Here's how the part is built. I have some questions about the finished solid (model axes, mm). Face numbers are marked on the shaded views. A direction names the side the tool comes from. Round coordinates to 2 decimals unless told otherwise and drop trailing zeros. Loops run counter-clockwise (first coordinate to the right, second up) from the corner with the lowest first, then second, coordinate; pieces in that order, holes last. Notation, with made-up numbers: M -21,-26.75 L 18,-26.75 A23 cw 18,-13.75 Z; hole C 33.5,-3.5 d4. An arc over 180 degrees is marked long. One line per question, with ' | ' between items. Start each with the question number.
```python
from build123d import *

# Parameters (mm, degrees)
BOSS_EXTRUDE1_DEPTH = 3
BOSS_EXTRUDE3_DEPTH = 3


with BuildPart() as part:
    # Sketch1 → Boss-Extrude1 (new body)
    with BuildSketch(Plane(origin=(0, 0, 0), x_dir=(1, 0, 0), z_dir=(0, 1, 0))):
        with BuildLine():
            Line((0, -6.1), (-30, -6.1))
            ThreePointArc((-30, -6.1), (-36.1, 0), (-30, 6.1))
            Line((-30, 6.1), (0, 6.1))
            Line((0, 6.1), (0, -6.1))
        make_face()
        with BuildLine():
            Line((-30, 3.1), (-25, 3.1))
            ThreePointArc((-25, 3.1), (-21.9, 0), (-25, -3.1))
            Line((-25, -3.1), (-30, -3.1))
            ThreePointArc((-30, -3.1), (-33.1, 0), (-30, 3.1))
        make_face(mode=Mode.SUBTRACT)
    extrude(amount=BOSS_EXTRUDE1_DEPTH)

    # Sketch4 → Boss-Extrude3 (add)
    with BuildSketch(Plane(origin=(0, 0, 0), x_dir=(0, 0, -1), z_dir=(1, 0, 0))):
        with BuildLine():
            Line((-6.1, 0), (-6.1, 30))
            ThreePointArc((-6.1, 30), (0, 36.1), (6.1, 30))
            Line((6.1, 30), (6.1, 0))
            Line((6.1, 0), (-6.1, 0))
        make_face()
        with BuildLine():
            Line((3.1, 30), (3.1, 25))
            ThreePointArc((3.1, 25), (0, 21.9), (-3.1, 25))
            Line((-3.1, 25), (-3.1, 30))
            ThreePointArc((-3.1, 30), (0, 33.1), (3.1, 30))
        make_face(mode=Mode.SUBTRACT)
    extrude(amount=-BOSS_EXTRUDE3_DEPTH)


solid = part.part
```
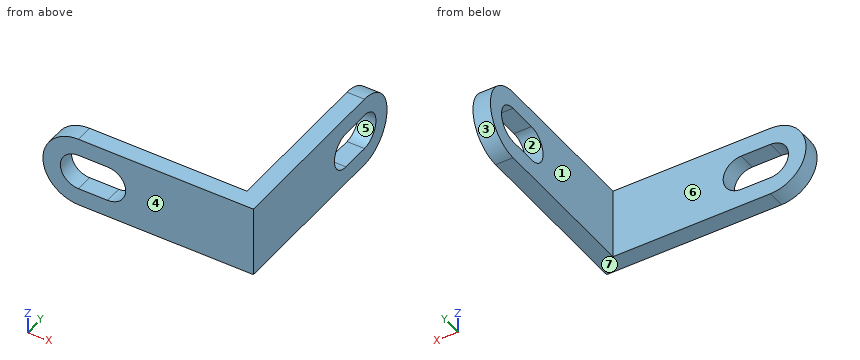
1) Please list where these lines run through material, in increasing order: L1, parallel to Y at x = -2.5, z = 0.25; L2, parallel to X at y = 21, z = 3; L3, parallel to Y at x = -6, z = 2.75. Write a range as from..to.
2) Imagine slicing it at D-D (y = 32.5). Write out the boundary of the cut face in (x, z).
3) We'd pull the mould along Y, two halves only. Please class the marked faces 1, 2, 3 and 4: pulls with the +Y half, pulls with the -Y half, needs draft (parallel to the pull), parting line crosses it, or undercut.
4) Imagine slicing it at C-C (z = 1.75). Write out the boundary of the cut face in (x, y), then the cut area to 3 significant figures.
5) Imagine slicing it at B-B (x = -29.5). Write out the boundary of the cut face in (y, z).
6) For the marked faces 5, 6 and 7, which set-ups out of +Z, -Z, +X, -X, +Y, -Y let a thin tool reach every point of the face, with its end or its side?
7) I'm going to push flat-ended pins straight in: pin 1 Ø1 at (x, y) = (-30.5, 5) entering from -Z; pin 2 Ø1 at (y, z) = (10.5, 4) entering from -X. Where does each tip first touch, or does it pass through?
8) Imagine slicing it at A-A (x = -2.5). Write out the boundary of the cut face in (y, z), then the cut area to 3 significant figures.
Results are:
1) L1: 0..21.91, 33.09..36.09 | L2: -3..0 | L3: 0..3
2) outline: M -3,-5.56 L 0,-5.56 L 0,-1.83 L -3,-1.83 Z; M -3,1.83 L 0,1.83 L 0,5.56 L -3,5.56 Z
3) face 1: needs draft | face 2: undercut | face 3: pulls with the +Y half | face 4: pulls with the -Y half
4) outline: M -35.84,0 L -32.56,0 L -32.56,3 L -35.84,3 Z; M -22.44,0 L 0,0 L 0,22.44 L -3,22.44 L -3,3 L -22.44,3 Z; M -3,32.56 L 0,32.56 L 0,35.84 L -3,35.84 Z | area: 145 mm²
5) outline: M 0,-6.1 L 3,-6.1 L 3,-3.1 L 0,-3.1 Z; M 0,3.1 L 3,3.1 L 3,6.1 L 0,6.1 Z
6) face 5: +X, -X | face 6: +Z, -Z, -X, +Y | face 7: -Z, +X, -X, +Y, -Y
7) pin 1: through | pin 2: x = -3
8) outline: M 0,-6.1 L 30,-6.1 A6.1 ccw 30,6.1 L 0,6.1 Z; hole M 25,-3.1 L 30,-3.1 A3.1 ccw 30,3.1 L 25,3.1 A3.1 ccw Z | area: 363 mm²
